CAD build for the part. Positions are in the model's coordinates, mm. Face numbers are marked on the shaded views. Round coordinates to 2 decimals unless told otherwise and drop trailing zeros. Write each loop counter-clockwise with the first axis right and the second up, starting at its lowest first coordinate (ties: lowest second). Pieces come first, ordered by that corner, then holes. Notation, with made-up numbers: (38, 44.5) -> (80, 44.5) arc R19 cw to (80, 73.5) -> close; hole circle Ø3 at (-15, 44). An arc over 180 degrees is marked (long way). Put each result on its own line as item: value. Start each with the question number.
1. Saw through at D-D on x = 9.5. List the corners of the cut face in (y, z).
2. Drill centre lines: line 1 (Y direction, x = 2, z = -3.25); line 2 (Z direction, x = 9.5, y = 1.35); line 3 (X direction, y = 0.95, z = -13). Where is each one in solid material? Low to high. Write a range as from..to.
3. Saw through at B-B on x = 17. List the corners of the cut face in (y, z), and give its area (3 significant figures).
4. Pull direction Y, two halves, no side cores. Call the marked faces 1, 2, 3 and 4: pulls with the +Y half, pulls with the -Y half, needs draft (parallel to the pull), parting line crosses it, or undercut.
5. Saw through at C-C on z = -7.5. List the corners of the cut face in (x, y).
6. Saw through at A-A on y = 2. List the corners of the cut face in (x, z), and give its area (3 significant figures).
7. Flat gauge pin, fed straight in: P1, Ø1.5, axis at y = 1.5, z = -12, coming from the -X side. Where does the tip first touch, or does it go through?
from build123d import *

# Parameters (mm, degrees)
SKETCH1_W           = 19
SKETCH1_H           = 15
SKETCH1_R           = 5.25
BOSS_EXTRUDE1_DEPTH = 4
SKETCH2_R           = 1.5
CUT_EXTRUDE1_DEPTH  = 15


with BuildPart() as part:
    # Sketch1 → Boss-Extrude1 (new body)
    with BuildSketch(Plane(origin=(0, 0, 0), x_dir=(1, 0, 0), z_dir=(0, 1, 0))):
        with Locations((9.5, 7.5)):
            Rectangle(SKETCH1_W, SKETCH1_H)
        with Locations((9.5, 7.5)):
            Circle(SKETCH1_R, mode=Mode.SUBTRACT)
    extrude(amount=BOSS_EXTRUDE1_DEPTH)

    # Sketch2 → Cut-Extrude1 (cut)
    with BuildSketch(Plane.XY):
        with Locations((2, 2)):
            Circle(SKETCH2_R)
        with Locations((17, 2)):
            Circle(SKETCH2_R)
    extrude(amount=-CUT_EXTRUDE1_DEPTH, mode=Mode.SUBTRACT)


solid = part.part
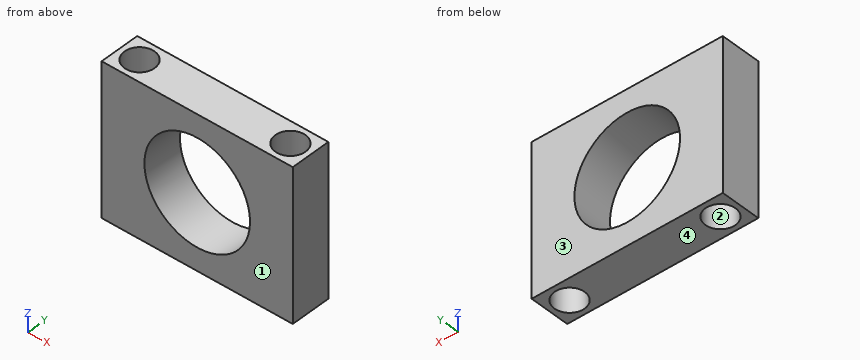
Return value:
1. outline: (0, -15) -> (4, -15) -> (4, -12.75) -> (0, -12.75) -> close; (0, -2.25) -> (4, -2.25) -> (4, 0) -> (0, 0) -> close
2. line 1: y = 0..0.5, 3.5..4
2. line 2: z = -15..-12.75, -2.25..0
2. line 3: x = 0..0.93, 3.07..15.93, 18.07..19
3. outline: (0, -15) -> (0.5, -15) -> (0.5, 0) -> (0, 0) -> close; (3.5, -15) -> (4, -15) -> (4, 0) -> (3.5, 0) -> close
3. area: 15.0 mm^2
4. face 1: pulls with the -Y half
4. face 2: undercut
4. face 3: pulls with the +Y half
4. face 4: needs draft
5. outline: (0, 0) -> (4.25, 0) -> (4.25, 4) -> (0, 4) -> close; (14.75, 0) -> (19, 0) -> (19, 4) -> (14.75, 4) -> close; hole circle Ø3 at (2, 2); hole circle Ø3 at (17, 2)
6. outline: (0, -15) -> (0.5, -15) -> (0.5, 0) -> (0, 0) -> close; (3.5, -15) -> (15.5, -15) -> (15.5, 0) -> (3.5, 0) -> close; (18.5, -15) -> (19, -15) -> (19, 0) -> (18.5, 0) -> close; hole circle Ø10.5 at (9.5, -7.5)
6. area: 108 mm^2
7. P1: stops at x = 0
